Model file for the job. Use its own axes, mm. Face numbers are marked on the shaded views. Coordinates: 2 decimals unless noted, no trailing zeros. Loops run counter-clockwise (first coordinate to the right, second up) from the corner with the lowest first, then second, coordinate; pieces in that order, holes last. Notation, with made-up numbers: (38, 37) -> (64, 37) arc R33 ccw to (64, 66) -> close; hole circle Ø10 at (13.5, -12). An arc over 180 degrees is marked (long way). Use one line per item in the form item = value.
```python
from build123d import *

# Parameters (mm, degrees)
SKETCH1_R           = 25
SKETCH1_R_2         = 5
SKETCH1_R_3         = 6
BOSS_EXTRUDE1_DEPTH = 10
SKETCH2_R           = 1
CUT_EXTRUDE1_DEPTH  = 15


with BuildPart() as part:
    # Sketch1 → Boss-Extrude1 (new body)
    with BuildSketch(Plane(origin=(0, 0, 0), x_dir=(0, 0, -1), z_dir=(1, 0, 0))):
        Circle(SKETCH1_R)
        with Locations((0, 18)):
            Circle(SKETCH1_R_2, mode=Mode.SUBTRACT)
        with Locations((12.727922061, 12.727922061)):
            Circle(SKETCH1_R_2, mode=Mode.SUBTRACT)
        with Locations((18, 0)):
            Circle(SKETCH1_R_2, mode=Mode.SUBTRACT)
        with Locations((12.727922061, -12.727922061)):
            Circle(SKETCH1_R_2, mode=Mode.SUBTRACT)
        with Locations((0, -18)):
            Circle(SKETCH1_R_2, mode=Mode.SUBTRACT)
        with Locations((-12.727922061, -12.727922061)):
            Circle(SKETCH1_R_2, mode=Mode.SUBTRACT)
        with Locations((-18, 0)):
            Circle(SKETCH1_R_2, mode=Mode.SUBTRACT)
        with Locations((-12.727922061, 12.727922061)):
            Circle(SKETCH1_R_2, mode=Mode.SUBTRACT)
        Circle(SKETCH1_R_3, mode=Mode.SUBTRACT)
    extrude(amount=BOSS_EXTRUDE1_DEPTH)

    # Sketch2 → Cut-Extrude1 (cut)
    with BuildSketch(Plane.ZY):
        with Locations((-9.265, 0)):
            Circle(SKETCH2_R)
        with Locations((9.265, 0)):
            Circle(SKETCH2_R)
    extrude(amount=-CUT_EXTRUDE1_DEPTH, mode=Mode.SUBTRACT)


solid = part.part
```
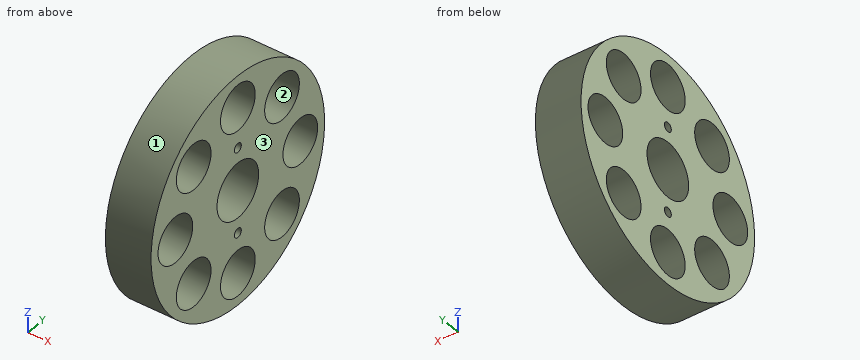
Q1. Band-saw the part on C-C, the plane y = -16. Write the cut outline in (x, z), and give its area (3 significant figures).
Result:
outline = (0, -19.21) -> (10, -19.21) -> (10, -16.51) -> (0, -16.51) -> close; (0, -8.95) -> (10, -8.95) -> (10, -4.58) -> (0, -4.58) -> close; (0, 4.58) -> (10, 4.58) -> (10, 8.95) -> (0, 8.95) -> close; (0, 16.51) -> (10, 16.51) -> (10, 19.21) -> (0, 19.21) -> close
area = 141 mm2
Q2. Band-saw the part on B-B, the plane z = 0. Write the cut outline in (x, y).
Result:
outline = (0, -25) -> (10, -25) -> (10, -23) -> (0, -23) -> close; (0, -13) -> (10, -13) -> (10, -6) -> (0, -6) -> close; (0, 6) -> (10, 6) -> (10, 13) -> (0, 13) -> close; (0, 23) -> (10, 23) -> (10, 25) -> (0, 25) -> close
Q3. Pin check, flat tips, straight feed: pin 1 Ø1.5 at (x, z) = (5.5, 4.5) entering from +Y; pin 2 Ø6 at (x, y) = (8.5, 13) entering from -Z; pin 3 Ø6 at (x, y) = (3, 9) entering from +Z. Stop position of each tip, or through.
Result:
pin_1 = 24.72
pin_2 = -22.91
pin_3 = 24.27
Q4. Mould opens along Y. For the marked faces 1, 2 and 3 say: released by +Y, released by -Y, zero draft, split by the parting line, or undercut.
Result:
face_1 = split by the parting line
face_2 = undercut
face_3 = zero draft
Q5. Band-saw the part on A-A, the plane y = 0. Write the cut outline in (x, z) (3 decimals).
Result:
outline = (0, -25) -> (10, -25) -> (10, -23) -> (0, -23) -> close; (0, -13) -> (10, -13) -> (10, -10.265) -> (0, -10.265) -> close; (0, -8.265) -> (10, -8.265) -> (10, -6) -> (0, -6) -> close; (0, 6) -> (10, 6) -> (10, 8.265) -> (0, 8.265) -> close; (0, 10.265) -> (10, 10.265) -> (10, 13) -> (0, 13) -> close; (0, 23) -> (10, 23) -> (10, 25) -> (0, 25) -> close
Q6. Wall check: line 1 along Y through (x, z) = (2.5, 0); line 2 along Z through (x, y) = (1.25, -11); line 3 along Z through (x, y) = (0.5, -16). Give the ranges that are in metal, low to high.
Result:
line_1 = -25 to -23, -13 to -6, 6 to 13, 23 to 25
line_2 = -22.45 to -17.42, -8.04 to 8.04, 17.42 to 22.45
line_3 = -19.21 to -16.51, -8.95 to -4.58, 4.58 to 8.95, 16.51 to 19.21
Q7. Band-saw the part on D-D, the plane x = 7. State how many separate pieces and enclosed holes the cut face has, and give its area (3 significant figures).
Result:
separate_pieces = 1
enclosed_holes = 11
area = 1,220 mm2
